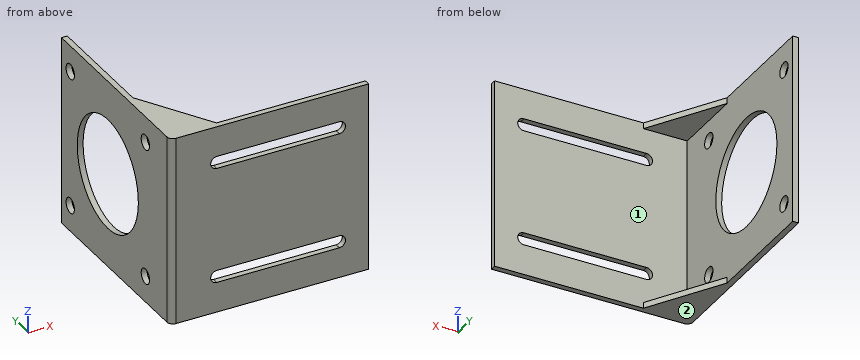
```python
from build123d import *

# Parameters (mm, degrees)
EXTRUDE_1_DEPTH     = 65
SKETCH_2_R          = 19.1
SKETCH_2_R_2        = 2.6
CUT_EXTRUDE_1_DEPTH = 3
CUT_EXTRUDE_2_DEPTH = 3
EXTRUDE_2_DEPTH     = 2
EXTRUDE_3_DEPTH     = 2


with BuildPart() as part:
    # Эскиз1 → Бобышка-Вытянуть1 (new body)
    with BuildSketch(Plane.XY):
        with BuildLine():
            Line((2, 0), (68, 0))
            Line((68, 0), (68, 2))
            Line((68, 2), (2, 2))
            Line((2, 2), (2, 68))
            Line((2, 68), (0, 68))
            Line((0, 68), (0, 2))
            ThreePointArc((0, 2), (0.585786438, 0.585786438), (2, 0))
        make_face()
    extrude(amount=EXTRUDE_1_DEPTH)

    # Эскиз2 → Вырез-Вытянуть1 (cut, through all)
    with BuildSketch(Plane(origin=(2, 0, 0), x_dir=(0, 0, -1), z_dir=(1, 0, 0))):
        with Locations((-32.5, 39)):
            Circle(SKETCH_2_R)
        with Locations((-9, 62.5)):
            Circle(SKETCH_2_R_2)
        with Locations((-9, 15.5)):
            Circle(SKETCH_2_R_2)
        with Locations((-56, 15.5)):
            Circle(SKETCH_2_R_2)
        with Locations((-56, 62.5)):
            Circle(SKETCH_2_R_2)
    extrude(amount=-CUT_EXTRUDE_1_DEPTH, mode=Mode.SUBTRACT)

    # Эскиз3 → Вырез-Вытянуть2 (cut, through all)
    with BuildSketch(Plane(origin=(0, 2, 0), x_dir=(1, 0, 0), z_dir=(0, 1, 0))):
        with BuildLine():
            Line((16, -10.4), (58, -10.4))
            ThreePointArc((58, -10.4), (60.1, -12.5), (58, -14.6))
            Line((58, -14.6), (16, -14.6))
            ThreePointArc((16, -14.6), (13.9, -12.5), (16, -10.4))
        make_face()
        with BuildLine():
            Line((16, -50.4), (58, -50.4))
            ThreePointArc((58, -50.4), (60.1, -52.5), (58, -54.6))
            Line((58, -54.6), (16, -54.6))
            ThreePointArc((16, -54.6), (13.9, -52.5), (16, -50.4))
        make_face()
    extrude(amount=-CUT_EXTRUDE_2_DEPTH, mode=Mode.SUBTRACT)

    # Эскиз4 → Бобышка-Вытянуть2 (add)
    with BuildSketch(Plane.XY.offset(65)):
        Polygon((2, 27), (17, 2), (2, 2), align=None)
    extrude(amount=-EXTRUDE_2_DEPTH)

    # Эскиз5 → Бобышка-Вытянуть3 (add)
    with BuildSketch(Plane(origin=(0, 0, 0), x_dir=(-1, 0, 0), z_dir=(0, 0, -1))):
        Polygon((-2, 27), (-17, 2), (-2, 2), align=None)
    extrude(amount=-EXTRUDE_3_DEPTH)


solid = part.part
```
Here's how the part is built. I have some questions about the finished solid (model axes, mm). Face numbers are marked on the shaded views. A direction names the side the tool comes from. Give positions to 0.01 mm unless a question says otherwise; leave off trailing zeros. Loops run counter-clockwise (first coordinate to the right, second up) from the corner with the lowest first, then second, coordinate; pieces in that order, holes last. Notation, with made-up numbers: M 2,54 L 16,54 A17 ccw 16,84 Z; hole C 88,-4 d7. An arc over 180 degrees is marked long. Return JSON: item names as keys, results as strings.
Item 1: Imagine slicing it at A-A on y = 15.5. List the corners of the cut face in (x, z) for me, then the cut area to 3 significant figures.
A:
{"outline": "M 0,0 L 8.9,0 L 8.9,2 L 2,2 L 2,6.4 L 0,6.4 Z; M 0,11.6 L 2,11.6 L 2,53.4 L 0,53.4 Z; M 0,58.6 L 2,58.6 L 2,63 L 8.9,63 L 8.9,65 L 0,65 Z", "area": "137 mm^2"}
Item 2: Please list where these lines run through material, in increasing order: line 1 (Z direction, x = 1, y = 62); line 2 (Y direction, x = 1, z = 9); line 3 (X direction, y = 30.5, z = 54.5).
A:
{"line 1": "z = 0 to 6.45, 11.55 to 53.45, 58.55 to 65", "line 2": "y = 0.27 to 12.9, 18.1 to 59.9, 65.1 to 68", "line 3": "x = 0 to 2"}
Item 3: I'm going to push flat-ended pins straight in: pin 1 Ø8.5 at (y, z) = (62.5, 9) entering from +X; pin 2 Ø1 at (x, z) = (17.5, 26) entering from -Y; pin 3 Ø2 at (x, z) = (18, 8) entering from +Y. Where does each tip first touch, or does it pass through?
A:
{"pin 1": "stops at x = 2", "pin 2": "stops at y = 0", "pin 3": "stops at y = 2"}
Item 4: On a 3-axis mill with a long thin cutter (end or side, diameter ignored), from which of +Z, -Z, +X, -X, +Y, -Y can I reach the whole of each face in a straight line? I mean the marked faces 1 and 2. Say none if no direction works.
A:
{"face 1": "+X, +Y", "face 2": "-Z, +X, -X, +Y, -Y"}
Item 5: Imagine slicing it at B-B on x = 38. List the corners of the cut face in (y, z) for me, then the cut area to 3 significant figures.
A:
{"outline": "M 0,0 L 2,0 L 2,10.4 L 0,10.4 Z; M 0,14.6 L 2,14.6 L 2,50.4 L 0,50.4 Z; M 0,54.6 L 2,54.6 L 2,65 L 0,65 Z", "area": "113 mm^2"}
Item 6: Imagine slicing it at D-D on y = 39. List the corners of the cut face in (x, z) for me.
A:
{"outline": "M 0,0 L 2,0 L 2,13.4 L 0,13.4 Z; M 0,51.6 L 2,51.6 L 2,65 L 0,65 Z"}
Item 7: Imagine slicing it at C-C on z = 32.5. List the corners of the cut face in (x, y) for me.
A:
{"outline": "M 0,2 A2 ccw 2,0 L 68,0 L 68,2 L 2,2 L 2,19.9 L 0,19.9 Z; M 0,58.1 L 2,58.1 L 2,68 L 0,68 Z"}
